```python
from build123d import *

# Parameters (mm, degrees)
SKETCH1_W           = 12
SKETCH1_H           = 12
BOSS_EXTRUDE1_DEPTH = 10
BOSS_EXTRUDE2_DEPTH = 3
CHAMFER1_SIZE       = 1
SKETCH1_4_R         = 1.5
CUT_EXTRUDE1_DEPTH  = 15.711220208


with BuildPart() as part:
    # Sketch1 → Boss-Extrude1 (new body)
    with BuildSketch(Plane(origin=(0, 0, 0), x_dir=(1, 0, 0), z_dir=(0, 1, 0))):
        with Locations((-2.9, 0.1)):
            Rectangle(SKETCH1_W, SKETCH1_H)
    extrude(amount=-BOSS_EXTRUDE1_DEPTH)

    # Sketch1<3> → Boss-Extrude2 (add)
    with BuildSketch(Plane(origin=(0, 0, 0), x_dir=(1, 0, 0), z_dir=(0, 1, 0))):
        Polygon((0, 6.1), (0, 4.1), (-6.9, 4.1), (-6.9, 0), (-8.9, 0), (-8.9, 6.1), align=None)
    extrude(amount=BOSS_EXTRUDE2_DEPTH)

    # Chamfer1
    chamfer1_edges = [part.edges().sort_by_distance(p)[0] for p in [
        (-8.9, -3.5, -6.1),
        (3.1, -5, -6.1),
        (3.1, -5, 5.9),
        (-8.9, -5, 5.9),
    ]]
    chamfer(chamfer1_edges, length=CHAMFER1_SIZE)

    # Sketch1<4> → Cut-Extrude1 (cut, through all)
    with BuildSketch(Plane(origin=(0, 0, 0), x_dir=(1, 0, 0), z_dir=(0, 1, 0))):
        with Locations(Location((0, 0, 0), (0, 0, 270))):
            Circle(SKETCH1_4_R)
    extrude(amount=-CUT_EXTRUDE1_DEPTH, mode=Mode.SUBTRACT)


solid = part.part
```
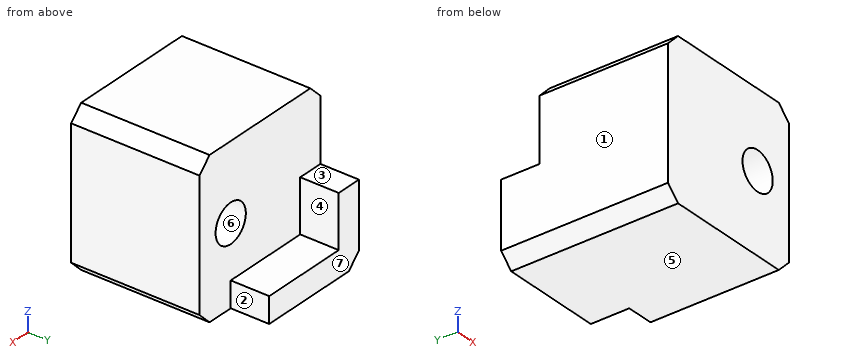
Work out the finished part from the listing and answer in its coordinate system (mm). Face numbers are marked on the shaded views. A direction names the side the tool comes from. Round coordinates to 2 decimals unless told otherwise and drop trailing zeros. Loops run counter-clockwise (first coordinate to the right, second up) from the corner with the lowest first, then second, coordinate; pieces in that order, holes last. Notation, with made-up numbers: (-18.5, -15) -> (19.5, -15) arc R11 ccw to (19.5, -3) -> close; hole circle Ø4 at (-19.5, 47). An arc over 180 degrees is marked (long way). Write each question's results on one line, items separated by ' | '. Start each with the question number.
1. A tool of negligible diameter and unlimited length cuts with its end or side. For the marked faces 1, 2, 3 and 4, from which of +Z, -Z, +X, -X, +Y, -Y can it reach the whole face along a straight path? Write none if from no direction.
2. Find the intervals of material crossed by probe 1 along X at (y, z) = (-2.25, 0); probe 2 along Y at (x, z) = (-7, 3.25); probe 3 along Z at (x, y) = (-0.5, -4.5), in increasing order. Write a range as from..to.
3. Section A-A (y = -1) is taken. Determine the outline of the cut face in (x, z).
4. For a pull along Z with two mould halves and no side action, classify the marked faces 5, 6 and 7 as +Z half, -Z half, draft (parallel to the pull), parting line (faces both ways), or undercut.
5. Section C-C (z = 4) is taken. Determine the outline of the cut face in (x, y), plus the area to 3 significant figures.
6. Given pin 1 Ø3.5 at (x, z) = (-3, -2) entering from +Y; pin 2 Ø2 at (x, y) = (-8, 2) entering from +Z; pin 3 Ø2.5 at (y, z) = (1.5, -1.5) entering from +X, each flat-ended and moving along its own axis, determine where each tip first touches the part or whether it passes through.
7. Section B-B (x = -4.75) is taken. Determine the outline of the cut face in (y, z).
Evaluation:
1) face 1: +Z, -Z, -X, +Y, -Y | face 2: +Z, -Z, +X, +Y | face 3: +Z, +X, -X, +Y | face 4: +Z, +X, +Y
2) probe 1: x = -8.9..-1.5, 1.5..3.1 | probe 2: y = -10..0 | probe 3: z = -6.1..-1.41, 1.41..5.9
3) outline: (-8.9, -5.1) -> (-7.9, -6.1) -> (2.1, -6.1) -> (3.1, -5.1) -> (3.1, 4.9) -> (2.1, 5.9) -> (-7.9, 5.9) -> (-8.9, 4.9) -> close; hole circle Ø3 at (0, 0)
4) face 5: -Z half | face 6: undercut | face 7: draft
5) outline: (-8.9, -10) -> (3.1, -10) -> (3.1, 0) -> (-8.9, 0) -> close | area: 120 mm2
6) pin 1: stops at y = 0 | pin 2: stops at z = 0 | pin 3: stops at x = -6.9
7) outline: (-10, -6.1) -> (3, -6.1) -> (3, -4.1) -> (0, -4.1) -> (0, 5.9) -> (-10, 5.9) -> close
